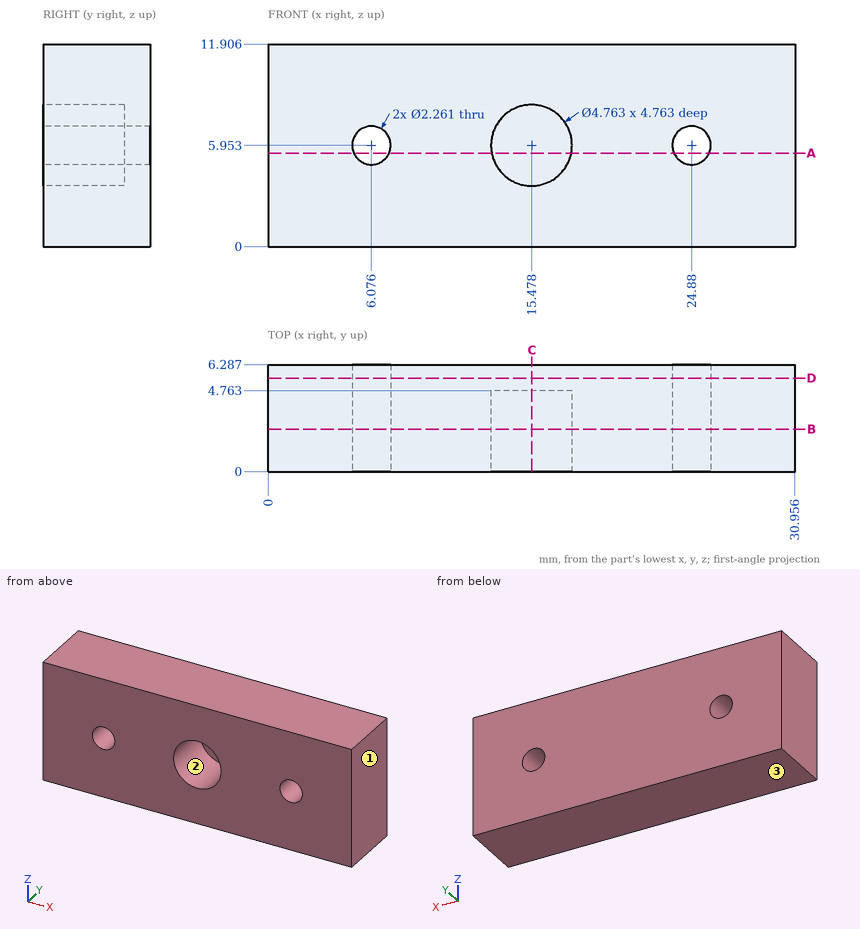
For this review, use the dimensioned drawing (mm, ordinates from the lowest corner) and the shaded views. Coordinates: 2 decimals unless noted, no trailing zeros. Loops run counter-clockwise (first coordinate to the right, second up) from the corner with the lowest first, then second, coordinate; pieces in that order, holes last.
1. Add section A-A, the plane z = 5.5. Give the boundary of the cut face in (x, y) (1 decimal).
2. Add section B-B, the plane y = 2.5. Give the boundary of the cut face in (x, z), then the cut area to 3 significant figures.
3. Add section C-C, the plane x = 15.5. Give the boundary of the cut face in (y, z) (1 decimal).
4. Mouldability with a two-part tool opening along X and no side actions: class the marked faces 1, 2 and 3 as +X half, -X half, draft (parallel to the pull), parting line (faces both ways), or undercut.
5. Add section D-D, the plane y = 5.5. Give the boundary of the cut face in (x, z).
6. For line 1 (X direction, y = 1.75, z = 6.25) (1 decimal); line 2 (Z direction, x = 13.5, y = 2.5) (1 decimal); line 3 (X direction, y = 2, z = 4.5) (1 decimal), list the stretches that pass through material, from the lowest coordinate up.
Result:
1. outline: (0, 0) - (5, 0) - (5, 6.3) - (0, 6.3) - close; (7.1, 0) - (13.1, 0) - (13.1, 4.8) - (17.8, 4.8) - (17.8, 0) - (23.8, 0) - (23.8, 6.3) - (7.1, 6.3) - close; (25.9, 0) - (31, 0) - (31, 6.3) - (25.9, 6.3) - close
2. outline: (0, 0) - (30.96, 0) - (30.96, 11.91) - (0, 11.91) - close; hole circle Ø2.26 at (6.08, 5.95); hole circle Ø4.76 at (15.48, 5.95); hole circle Ø2.26 at (24.88, 5.95)
2. area: 343 mm2
3. outline: (0, 0) - (6.3, 0) - (6.3, 11.9) - (0, 11.9) - (0, 8.3) - (4.8, 8.3) - (4.8, 3.6) - (0, 3.6) - close
4. face 1: +X half
4. face 2: undercut
4. face 3: draft
5. outline: (0, 0) - (30.96, 0) - (30.96, 11.91) - (0, 11.91) - close; hole circle Ø2.26 at (6.08, 5.95); hole circle Ø2.26 at (24.88, 5.95)
6. line 1: x = 0 to 5, 7.2 to 13.1, 17.8 to 23.8, 26 to 31
6. line 2: z = 0 to 4.6, 7.3 to 11.9
6. line 3: x = 0 to 13.6, 17.4 to 31
